Verification items for this drawing (mm, ordinates from the low corner). Round coordinates to 2 decimals unless told otherwise and drop trailing zeros. Order: outer loops, then holes, each group sorted by start corner. A loop starts at its lowest first (then second) coordinate and runs counter-clockwise, first axis right, second up. Notation, with made-up numbers: (2, -1.5) - (47, -1.5) arc R32 ccw to (47, 27.5) - close; hole circle Ø5 at (-29.5, -25.75). An arc over 180 degrees is marked (long way). One line per question, with ' | ' between items. Start each with the question number.
Q1. Gauge pin test, flat ends, axial feed: P1, Ø1, axis at x = 0.5, z = 6, coming from the +Y side; P2, Ø1, axis at y = 0.5, z = 2.5, coming from the -X side; P3, Ø1.5, axis at x = 2.5, z = 6.5, coming from the -Y side; P4, Ø1, axis at y = 1, z = 6.5, coming from the -X side. Record the tip position at first contact, or that the pin passes through.
Q2. Mould release check, pull along Y, two halves, no side actions. Record for the marked faces 1, 2 and 3: +Y half, -Y half, draft (parallel to the pull), parting line (faces both ways), or undercut.
Q3. Sectioned sample at B-B, the plane z = 7.25. Enter the section's corners in (x, y), then the cut area to 3 significant figures.
Q4. Sectioned sample at D-D, the plane z = 4. Enter the section's corners in (x, y), then the cut area to 3 significant figures.
Q5. Sectioned sample at A-A, the plane x = 1.5. Enter the section's corners in (y, z), then the cut area to 3 significant figures.
Q6. Material ranges on line 1 along Y through (x, z) = (2.15, 2.5); line 2 along Y through (x, z) = (1.5, 7.75), recorded low to high.
Q7. Sectioned sample at C-C, the plane y = 1.5. Enter the section's corners in (x, z), then the cut area to 3 significant figures.
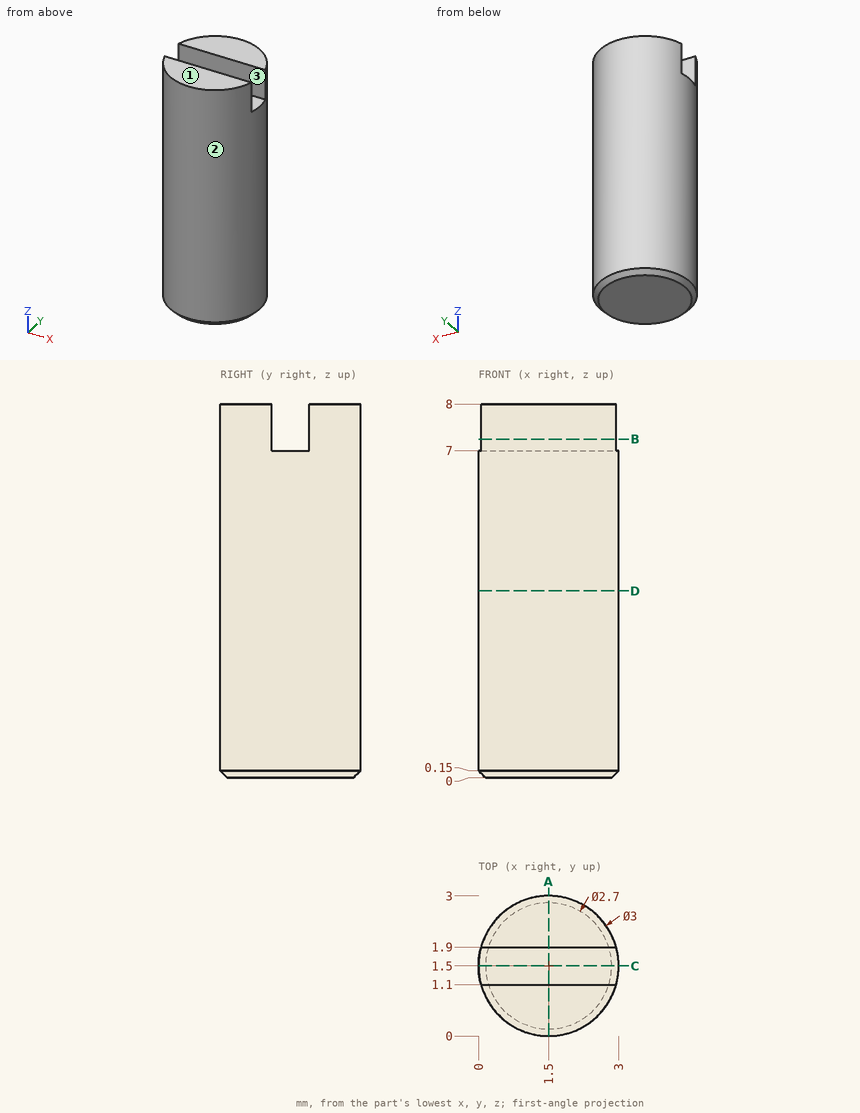
Determined:
1) P1: stops at y = 2.91 | P2: stops at x = 0.09 | P3: stops at y = 0.02 | P4: stops at x = 0
2) face 1: draft | face 2: parting line | face 3: undercut
3) outline: (0.05, 1.1) arc R1.5 ccw to (2.95, 1.1) - close; (0.05, 1.9) - (2.95, 1.9) arc R1.5 ccw to start | area: 4.70 mm2
4) outline: circle Ø3 at (1.5, 1.5) | area: 7.07 mm2
5) outline: (0, 0.15) - (0.15, 0) - (2.85, 0) - (3, 0.15) - (3, 8) - (1.9, 8) - (1.9, 7) - (1.1, 7) - (1.1, 8) - (0, 8) - close | area: 23.2 mm2
6) line 1: y = 0.15 to 2.85 | line 2: y = 0 to 1.1, 1.9 to 3
7) outline: (0, 0.15) - (0.15, 0) - (2.85, 0) - (3, 0.15) - (3, 7) - (0, 7) - close | area: 21.0 mm2
